from build123d import *

# Parameters (mm, degrees)
BOSS_EXTRUDE1_DEPTH     = 160
CUT_EXTRUDE1_DEPTH      = 305.764548692
CUT_EXTRUDE1_DEPTH_BACK = 305.764548692
BOSS_EXTRUDE2_DEPTH     = 20
SKETCH5_W               = 151.467001677
SKETCH5_H               = 170
CUT_EXTRUDE2_DEPTH      = 180
FILLET1_START           = -7.935101665
FILLET1_DEPTH           = 20.924834967
FILLET1_START_2         = 12.989733302
FILLET1_2_DEPTH         = 11.975549634
SKETCH6_R               = 5
SKETCH6_R_2             = 3.25
CUT_EXTRUDE3_DEPTH      = 180
CUT_EXTRUDE4_DEPTH      = 150
FILLET2_R               = 5


with BuildPart() as part:
    # Sketch1 → Boss-Extrude1 (new body)
    with BuildSketch(Plane.XY):
        Polygon((-67.312693498, 90.077399381), (130.687306502, 90.077399381), (133.687306502, 87.077399381), (133.687306502, 80.077399381), (136.687306502, 77.077399381), (143.687306502, 77.077399381), (146.687306502, 74.077399381), (146.687306502, -24.922600619), (131.687306502, -119.922600619), (-68.312693498, -119.922600619), (-83.312693498, -24.922600619), (-83.312693498, 74.077399381), (-80.312693498, 77.077399381), (-73.312693498, 77.077399381), (-70.312693498, 80.077399381), (-70.312693498, 87.077399381), align=None)
    extrude(amount=BOSS_EXTRUDE1_DEPTH)

    # Sketch4 → Cut-Extrude1 (cut, two sides: drawn at the far end of the back side and taken through both)
    with BuildSketch(Plane(origin=(146.687306502, 0, 0), x_dir=(0, 0, -1), z_dir=(1, 0, 0)).offset(-CUT_EXTRUDE1_DEPTH_BACK)):
        Polygon((533.86053197, -186.655167115), (0, -119.922600619), (-160, -99.922600619), (-693.86053197, -33.190034123), (-827.325664962, -1100.911098062), (400.395398977, -1254.376231054), align=None)
    extrude(amount=CUT_EXTRUDE1_DEPTH + CUT_EXTRUDE1_DEPTH_BACK, mode=Mode.SUBTRACT)

    # 3DSketch1 → Boss-Extrude2 (add, along a direction that is not the sketch's normal)
    with BuildSketch(Plane(origin=(-55.046194337, -112.922600619, 0), x_dir=(0.6840030395475861, 0.727675877553092, -0.05126069758597554), z_dir=(0, 0.07027027027027033, 0.9975279891392237))):
        Polygon((0, 0), (118.651956408, -126.540562316), (253.60560063, 0), (134.953644222, 126.540562316), align=None)
    extrude(amount=BOSS_EXTRUDE2_DEPTH, dir=(0, 0, 1))

    # Sketch5 → Cut-Extrude2 (cut)
    with BuildSketch(Plane(origin=(0, -0.557601739, -7.915486008), x_dir=(-1, 0, 0), z_dir=(0, -0.07027027027027048, -0.9975279891392237))):
        with Locations((-31.687306502, -20.143454724)):
            Rectangle(SKETCH5_W, SKETCH5_H)
    extrude(amount=-CUT_EXTRUDE2_DEPTH, mode=Mode.SUBTRACT)

    # Fillet1: read off the stored shape, not the designer's step
    # Fillet1 outline → Fillet1 (add)
    with BuildSketch(Plane(origin=(0, 0, 0), x_dir=(1, 0, 0), z_dir=(0, 0.07027027027027048, 0.9975279891392238)).offset(FILLET1_START)):
        with BuildLine():
            ThreePointArc((107.42080734, -95.143454724), (104.491875152, -102.214522536), (97.42080734, -105.143454724))
            Line((97.42080734, -105.143454724), (107.42080734, -105.143454724))
            Line((107.42080734, -105.143454724), (107.42080734, -95.143454724))
        make_face()
        with BuildLine():
            Line((-44.046194337, -105.143454724), (-34.046194337, -105.143454724))
            ThreePointArc((-34.046194337, -105.143454724), (-41.117262149, -102.214522536), (-44.046194337, -95.143454724))
            Line((-44.046194337, -95.143454724), (-44.046194337, -105.143454724))
        make_face()
        with BuildLine():
            ThreePointArc((97.42080734, 64.856545276), (104.491875152, 61.927613088), (107.42080734, 54.856545276))
            Line((107.42080734, 54.856545276), (107.42080734, 64.856545276))
            Line((107.42080734, 64.856545276), (97.42080734, 64.856545276))
        make_face()
        with BuildLine():
            Line((-44.046194337, 64.856545276), (-44.046194337, 54.856545276))
            ThreePointArc((-44.046194337, 54.856545276), (-41.117262149, 61.927613088), (-34.046194337, 64.856545276))
            Line((-34.046194337, 64.856545276), (-44.046194337, 64.856545276))
        make_face()
    extrude(amount=FILLET1_DEPTH)

    # Fillet1 2 outline → Fillet1 2 (add)
    with BuildSketch(Plane(origin=(0, 0, 0), x_dir=(1, 0, 0), z_dir=(0, 0.07027027027027048, 0.9975279891392238)).offset(FILLET1_START_2)):
        with BuildLine():
            ThreePointArc((97.42080734, 64.856545276), (104.491875152, 61.927613088), (107.42080734, 54.856545276))
            Line((107.42080734, 54.856545276), (107.42080734, 64.856545276))
            Line((107.42080734, 64.856545276), (97.42080734, 64.856545276))
        make_face()
        with BuildLine():
            Line((-44.046194337, 64.856545276), (-44.046194337, 54.856545276))
            ThreePointArc((-44.046194337, 54.856545276), (-41.117262149, 61.927613088), (-34.046194337, 64.856545276))
            Line((-34.046194337, 64.856545276), (-44.046194337, 64.856545276))
        make_face()
    extrude(amount=FILLET1_2_DEPTH)

    # Sketch6 → Cut-Extrude3 (cut)
    with BuildSketch(Plane(origin=(0, 0, 0), x_dir=(-1, 0, 0), z_dir=(0, 0, -1))):
        with Locations((-129.687306502, 57.077399381)):
            Circle(SKETCH6_R)
        with Locations((-129.687306502, 10.077399381)):
            Circle(SKETCH6_R)
        with Locations((66.312693498, 57.077399381)):
            Circle(SKETCH6_R)
        with Locations((66.312693498, 10.077399381)):
            Circle(SKETCH6_R_2)
        with Locations((66.312693498, -12.922600619)):
            Circle(SKETCH6_R)
    extrude(amount=-CUT_EXTRUDE3_DEPTH, mode=Mode.SUBTRACT)

    # Sketch7 → Cut-Extrude4 (cut)
    with BuildSketch(Plane.XY.offset(160)):
        Polygon((-75.312693498, 69.077399381), (-52.046194337, 69.077399381), (-52.046194337, -25.922600619), (-52.046194337, -92.030689236), (-63.956851508, -92.030689236), (-75.312693498, -27.22448539), align=None)
        Polygon((139.154308179, 69.077399381), (115.887809017, 69.077399381), (115.887809017, -25.922600619), (115.887809017, -92.030689236), (127.798466188, -92.030689236), (139.154308179, -27.22448539), align=None)
    extrude(amount=-CUT_EXTRUDE4_DEPTH, mode=Mode.SUBTRACT)

    # Fillet2
    fillet2_edges = [part.edges().sort_by_distance(p)[0] for p in [
        (-69.891640867, -109.922600619, 80),
        (133.26625387, -109.922600619, 80),
    ]]
    fillet(fillet2_edges, radius=FILLET2_R)


solid = part.part
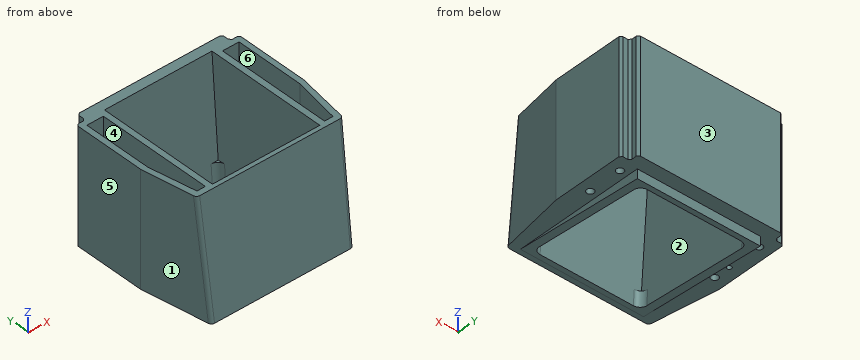
The model under review builds one solid part; all positions refer to its coordinate system, in mm. Face numbers are marked on the shaded views. A direction names the side the tool comes from. Round coordinates to 2 decimals unless told otherwise and drop trailing zeros. Order: outer loops, then holes, each group sorted by start corner. A loop starts at its lowest first (then second) coordinate and runs counter-clockwise, first axis right, second up. Notation, with made-up numbers: (-7, -12.5) -> (10, -12.5) arc R17 ccw to (10, -8.5) -> close; hole circle Ø8 at (88.25, 87.5). An arc over 180 degrees is marked (long way). Return JSON: item names as keys, results as strings.
1. For the marked faces 5 and 6, list the 3-axis set-ups (+Z, -Z, +X, -X, +Y, -Y) from which the entire face can be reached by the end or side of a thin tool; tool diameter is ignored.
Answer block:
{"face 5": "+Z, -Z, -X, +Y, -Y", "face 6": "+Z"}
2. Take a section at C-C (y = -76.5). Write out the cut boundary in (x, z).
Answer block:
{"outline": "(-75.17, 0) -> (-55.05, 0) -> (-55.05, -2.57) -> (-44.05, -2.57) -> (-44.05, 160) -> (-52.05, 160) -> (-52.05, 10) -> (-66.68, 10) -> (-66.68, 160) -> (-75.17, 160) -> close; (107.42, -2.57) -> (118.42, -2.57) -> (118.42, 0) -> (138.54, 0) -> (138.54, 160) -> (130.52, 160) -> (130.52, 10) -> (115.89, 10) -> (115.89, 160) -> (107.42, 160) -> close"}
3. Take a section at B-B (y = 36). Write out the cut boundary in (x, z), then the cut area to 3 significant figures.
Answer block:
{"outline": "(-83.31, 0) -> (-55.05, 0) -> (-55.05, -10.49) -> (-44.05, -10.49) -> (-44.05, 160) -> (-52.05, 160) -> (-52.05, 10) -> (-75.31, 10) -> (-75.31, 160) -> (-83.31, 160) -> close; (107.42, -10.49) -> (118.42, -10.49) -> (118.42, 0) -> (146.69, 0) -> (146.69, 160) -> (139.15, 160) -> (139.15, 10) -> (115.89, 10) -> (115.89, 160) -> (107.42, 160) -> close", "area": "5,820 mm²"}
4. Take a section at A-A (x = 92). Write out the cut boundary in (y, z).
Answer block:
{"outline": "(-119.92, 0) -> (-112.92, 0) -> (-105.44, -0.53) -> (-94.13, 160) -> (-99.92, 160) -> close; (64.14, -12.47) -> (71.62, -13) -> (71.62, 0) -> (90.08, 0) -> (90.08, 160) -> (76.29, 160) -> close"}
5. Insertion check: P1, Ø11.5, axis at x = 133, y = -27.5, coming from the +Z side; P2, Ø5, axis at x = 30.5, z = 22.5, coming from the -Y side; P3, Ø5.5, axis at x = -76.5, z = 105.5, coming from the +Y side. Each pin has a flat end and moves straight along its axis. Give the tip position at first contact, or say it passes through.
Answer block:
{"P1": "stops at z = 10", "P2": "stops at y = -117.42", "P3": "stops at y = 77.08"}
6. For L1, parallel to X at y = 4.5, z = 56; L2, parallel to X at y = -92, z = 149; L3, parallel to Z at x = -74, y = 71, list the stretches that pass through material, from the lowest coordinate up. Write a range as [from, to].
Answer block:
{"L1": "x = [-83.31, -75.31], [-52.05, -44.05], [107.42, 115.89], [139.15, 146.69]", "L2": "x = [-72.72, -63.96], [-52.05, -44.05], [107.42, 115.89], [127.8, 136.1]", "L3": "z = [0, 160]"}
7. The part is to be moulded in two halves that separate along Y. For the marked faces 1, 2, 3 and 4, say which applies: +Y half, -Y half, draft (parallel to the pull), parting line (faces both ways), or undercut.
Answer block:
{"face 1": "-Y half", "face 2": "undercut", "face 3": "+Y half", "face 4": "undercut"}
8. Take a section at D-D (z = 146). State how many separate pieces and enclosed holes the cut face has, then the cut area to 3 significant figures.
Answer block:
{"separate pieces": "1", "enclosed holes": "3", "area": "10,200 mm²"}
